from build123d import *

# Parameters (mm, degrees)
SKETCH_1_W          = 30
SKETCH_1_H          = 30
EXTRUDE_1_DEPTH     = 110
SKETCH_2_R          = 4
SKETCH_2_W          = 4
SKETCH_2_H          = 4
CUT_EXTRUDE_1_DEPTH = 113.026782512
FILLET_2_R          = 1


with BuildPart() as part:
    # 草图1 → 凸台-拉伸1 (new body)
    with BuildSketch(Plane.XY):
        Rectangle(SKETCH_1_W, SKETCH_1_H)
    extrude(amount=EXTRUDE_1_DEPTH)

    # 草图2 → 切除-拉伸1 (cut, through all)
    with BuildSketch(Plane.XY.offset(110)):
        Circle(SKETCH_2_R)
        Polygon((-8, 9.414213562), (-3.585786438, 5), (3.585786438, 5), (8, 9.414213562), (8, 13), (2.735613527, 13), (2.735613527, 15), (-2.735613527, 15), (-2.735613527, 13), (-8, 13), align=None)
        Polygon((-5, -3.585786438), (-5, 3.585786438), (-9.414213562, 8), (-13, 8), (-13, 2.735613527), (-15, 2.735613527), (-15, -2.735613527), (-13, -2.735613527), (-13, -8), (-9.414213562, -8), align=None)
        Polygon((3.585786438, -5), (-3.585786438, -5), (-8, -9.414213562), (-8, -13), (-2.735613527, -13), (-2.735613527, -15), (2.735613527, -15), (2.735613527, -13), (8, -13), (8, -9.414213562), align=None)
        Polygon((9.414213562, 8), (5, 3.585786438), (5, -3.585786438), (9.414213562, -8), (13, -8), (13, -2.735613527), (15, -2.735613527), (15, 2.735613527), (13, 2.735613527), (13, 8), align=None)
        with Locations((-11, 11)):
            Rectangle(SKETCH_2_W, SKETCH_2_H)
        with Locations((11, 11)):
            Rectangle(SKETCH_2_W, SKETCH_2_H)
        with Locations((11, -11)):
            Rectangle(SKETCH_2_W, SKETCH_2_H)
        with Locations((-11, -11)):
            Rectangle(SKETCH_2_W, SKETCH_2_H)
    extrude(amount=-CUT_EXTRUDE_1_DEPTH, mode=Mode.SUBTRACT)

    # 圆角2
    fillet_2_edges = [part.edges().sort_by_distance(p)[0] for p in [
        (-15, 15, 55),
        (15, 15, 55),
        (15, -15, 55),
        (-15, -15, 55),
    ]]
    fillet(fillet_2_edges, radius=FILLET_2_R)


solid = part.part
Verification items for the finished model (mm, model axes). A direction names the side the tool comes from. Give positions to 0.01 mm unless a question says otherwise; leave off trailing zeros. Write each loop counter-clockwise with the first axis right and the second up, starting at its lowest first coordinate (ties: lowest second). Pieces come first, ordered by that corner, then holes.
(1) Material ranges on line 1 (X direction, y = -10.5, z = 33); line 2 (Y direction, x = 0, z = 23), recorded low to high.
(2) Cross-section at C-C (y = 11). Enter the section's corners in (x, z).
(3) Cross-section at A-A (y = 0). Enter the section's corners in (x, z).
(4) Mould release check, pull along X, two halves, no side actions. Record for faces 5 (the face through (15, -8, 54)), 6 (the face through (8, -15, 54)), 7 (the face through (-7.238, -5.824, 55.77)), 8 (the face through (13, -11, 56)): +X half, -X half, draft (parallel to the pull), parting line (faces both ways), or undercut.
(5) Cross-section at D-D (z = 97.5). State how many separate pieces and enclosed holes the cut face has, plus the area to 3 significant figures.
(6) Access from +Z, -Z, +X, -X, +Y, -Y to the whole of each face (thin tool, end or side, straight path). Record for faces 1 (the face through (-14, 2.736, 56)), 2 (the face through (15, 8, 54)), 3 (the face through (14, 2.736, 56)), 4 (the face through (-11, 13, 56)).
(7) Gauge pin test, flat end, axial feed: pin 1 (0.6 mm diameter, centred on x = -14.5, z = 34.5, fed in from -Y). Record the tip position at first contact, or that the pin passes through.
Worked out:
1. line 1: x = -15 to -13, -9 to -8, 8 to 9, 13 to 15
1. line 2: y = -5 to -4, 4 to 5
2. outline: (-15, 0) - (-13, 0) - (-13, 110) - (-15, 110) - close; (-9, 0) - (-8, 0) - (-8, 110) - (-9, 110) - close; (8, 0) - (9, 0) - (9, 110) - (8, 110) - close; (13, 0) - (15, 0) - (15, 110) - (13, 110) - close
3. outline: (-5, 0) - (-4, 0) - (-4, 110) - (-5, 110) - close; (4, 0) - (5, 0) - (5, 110) - (4, 110) - close
4. face 5: +X half
4. face 6: draft
4. face 7: undercut
4. face 8: undercut
5. separate pieces: 1
5. enclosed holes: 5
5. area: 307 mm2
6. face 1: +Z, -Z, -X
6. face 2: +Z, -Z, +X, +Y, -Y
6. face 3: +Z, -Z, +X
6. face 4: +Z, -Z
7. pin 1: stops at y = -14.98
